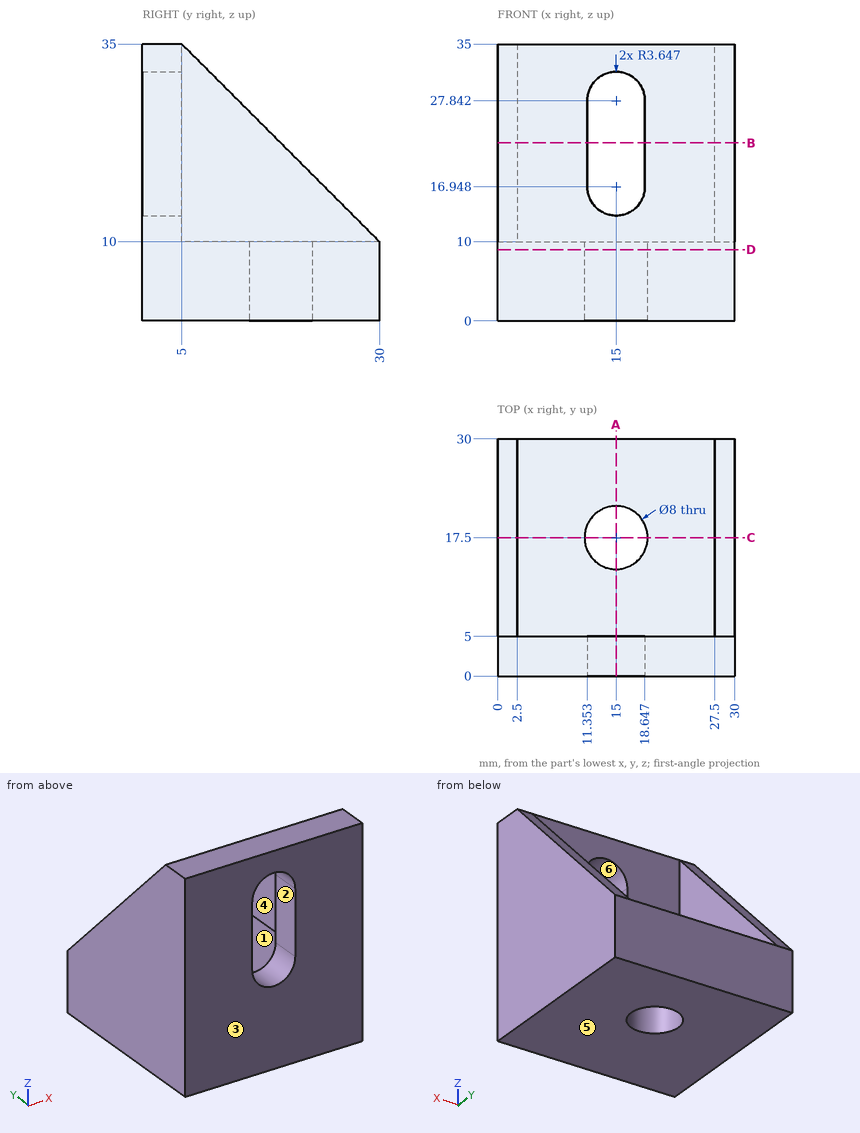
Input: dimensioned drawing with shaded views. Units: mm. Origin: part minimum x, y, z. A direction names the side the tool comes from. Give positions to 0.01 mm unless a question says otherwise; leave off trailing zeros. Loops run counter-clockwise (first coordinate to the right, second up) from the corner with the lowest first, then second, coordinate; pieces in that order, holes last. Notation, with made-up numbers: M 14,89.25 L 68,89.25 A30 cw 68,112.25 Z; hole C 25,-25 d5. An arc over 180 degrees is marked long. Put each result on its own line as item: value. Start each with the question number.
1) Cut plane A-A (x = 15). Output: boundary loops of the cut face in (y, z).
2) Contact query for flat-ended pins moving along their axis: pin 1 (3 mm diameter, centred on x = 21, y = 8.5, fed in from +Z); pin 2 (7.5 mm diameter, centred on x = 20, z = 22.5, fed in from +Y). Output: stop coordinate, or through.
3) Cut plane B-B (z = 22.5). Output: boundary loops of the cut face in (x, y).
4) Pull-direction query (Z, two-part tool) for the marked faces 4, 5 and 6; classes: pulls with the +Z half, pulls with the -Z half, needs draft (parallel to the pull), parting line crosses it, or undercut.
5) Cut plane D-D (z = 9). Output: boundary loops of the cut face in (x, y).
6) Cut plane C-C (y = 17.5). Output: boundary loops of the cut face in (x, z).
7) Ray query, line 1 along X through (y, z) = (8.5, 31); line 2 along Y through (x, z) = (15, 7.5); line 3 along Z through (x, y) = (8.25, 23.5). Return the intervals inside material, ascending.
8) Access query for the marked faces 1, 2 and 3. Directions: +Z, -Z, +X, -X, +Y, -Y. A direction counts if a zero-diameter tool reaches every point of the face in a straight line with its end or side. Return the directions, or none.
Verdict:
1. outline: M 0,0 L 13.5,0 L 13.5,10 L 5,10 L 5,13.3 L 0,13.3 Z; M 0,31.49 L 5,31.49 L 5,35 L 0,35 Z; M 21.5,0 L 30,0 L 30,10 L 21.5,10 Z
2. pin 1: z = 10
2. pin 2: y = 5
3. outline: M 0,0 L 11.35,0 L 11.35,5 L 2.5,5 L 2.5,17.5 L 0,17.5 Z; M 18.65,0 L 30,0 L 30,17.5 L 27.5,17.5 L 27.5,5 L 18.65,5 Z
4. face 4: needs draft
4. face 5: pulls with the -Z half
4. face 6: undercut
5. outline: M 0,0 L 30,0 L 30,30 L 0,30 Z; hole C 15,17.5 d8
6. outline: M 0,0 L 11,0 L 11,10 L 2.5,10 L 2.5,22.5 L 0,22.5 Z; M 19,0 L 30,0 L 30,22.5 L 27.5,22.5 L 27.5,10 L 19,10 Z
7. line 1: 0 to 2.5, 27.5 to 30
7. line 2: 0 to 13.5, 21.5 to 30
7. line 3: 0 to 10
8. face 1: +Z, +Y
8. face 2: +Y, -Y
8. face 3: +Z, -Z, +X, -X, -Y
